from build123d import *

# Parameters (mm, degrees)
SKETCH1_W           = 82.48
SKETCH1_H           = 33
BOSS_EXTRUDE1_DEPTH = 5
SKETCH2_W           = 82.48
SKETCH2_H           = 5
BOSS_EXTRUDE2_DEPTH = 5
CHAMFER1_SIZE       = 5
CUT_EXTRUDE1_REACH  = 92.95
SKETCH3_R           = 5.35
BOSS_EXTRUDE3_DEPTH = 22
SKETCH5_W           = 21.546115959
SKETCH5_H           = 2.75
SKETCH5_W_2         = 39.193884041
BOSS_EXTRUDE4_DEPTH = 15
SKETCH6_W           = 4
SKETCH6_H           = 23
BOSS_EXTRUDE5_DEPTH = 3
CUT_EXTRUDE2_REACH  = 95.44
SKETCH7_W           = 20.522158998
SKETCH7_H           = 19


with BuildPart() as part:
    # Sketch1 → Boss-Extrude1 (new body)
    with BuildSketch(Plane.XY):
        with Locations((41.24, 16.5)):
            Rectangle(SKETCH1_W, SKETCH1_H)
    extrude(amount=BOSS_EXTRUDE1_DEPTH)

    # Sketch2 → Boss-Extrude2 (add)
    with BuildSketch(Plane(origin=(0, 33, 0), x_dir=(1, 0, 0), z_dir=(0, 1, 0))):
        with Locations((41.24, -2.5)):
            Rectangle(SKETCH2_W, SKETCH2_H)
    extrude(amount=BOSS_EXTRUDE2_DEPTH)

    # Chamfer1
    chamfer1_edges = [part.edges().sort_by_distance(p)[0] for p in [
        (0, 38, 2.5),
        (82.48, 38, 2.5),
    ]]
    chamfer(chamfer1_edges, length=CHAMFER1_SIZE)

    # Sketch3 → Cut-Extrude1 (cut, up to next)
    with BuildSketch(Plane.XY.offset(5), mode=Mode.PRIVATE) as cut_extrude1_sk1:
        with Locations((62.98, 20)):
            Circle(SKETCH3_R)
    cut_extrude1_tool1 = extrude(cut_extrude1_sk1.sketch, amount=-CUT_EXTRUDE1_REACH, mode=Mode.PRIVATE) & part.part
    add(cut_extrude1_tool1.solids().sort_by_distance((62.98, 20, 5))[0], mode=Mode.SUBTRACT)

    # Sketch4 → Boss-Extrude3 (add)
    with BuildSketch(Plane(origin=(0, 0, 0), x_dir=(-1, 0, 0), z_dir=(0, 0, -1))):
        Polygon((-82.48, 33), (0, 33), (-5, 38), (-77.48, 38), align=None)
    extrude(amount=BOSS_EXTRUDE3_DEPTH)

    # Sketch5 → Boss-Extrude4 (add)
    with BuildSketch(Plane(origin=(0, 0, 0), x_dir=(-1, 0, 0), z_dir=(0, 0, -1))):
        Polygon((-79.23, 33), (-77.73, 33), (-77.73, 29.75), (-75.73, 29.75), (-75.73, 28.25), (-81.23, 28.25), (-81.23, 29.75), (-79.23, 29.75), align=None)
        Polygon((-6.49, 33), (-4.99, 33), (-4.99, 29.75), (-2.99, 29.75), (-2.99, 28.25), (-8.49, 28.25), (-8.49, 29.75), (-6.49, 29.75), align=None)
        with Locations((-68.456942021, 4.625)):
            Rectangle(SKETCH5_W, SKETCH5_H)
        with Locations((-22.586942021, 4.625)):
            Rectangle(SKETCH5_W_2, SKETCH5_H)
    extrude(amount=BOSS_EXTRUDE4_DEPTH)

    # Sketch6 → Boss-Extrude5 (add)
    with BuildSketch(Plane(origin=(0, 0, 0), x_dir=(-1, 0, 0), z_dir=(0, 0, -1))):
        with Locations((-49.262158998, 21.5)):
            Rectangle(SKETCH6_W, SKETCH6_H)
        with Locations((-38.262158998, 21.5)):
            Rectangle(SKETCH6_W, SKETCH6_H)
    extrude(amount=BOSS_EXTRUDE5_DEPTH)

    # Sketch7 → Cut-Extrude2 (cut, up to next)
    with BuildSketch(Plane(origin=(0, 0, 0), x_dir=(-1, 0, 0), z_dir=(0, 0, -1)), mode=Mode.PRIVATE) as cut_extrude2_sk1:
        with Locations((-19.751079499, 19.5)):
            Rectangle(SKETCH7_W, SKETCH7_H)
    cut_extrude2_tool1 = extrude(cut_extrude2_sk1.sketch, amount=-CUT_EXTRUDE2_REACH, mode=Mode.PRIVATE) & part.part
    add(cut_extrude2_tool1.solids().sort_by_distance((19.751079, 19.5, 0))[0], mode=Mode.SUBTRACT)


solid = part.part
Here's how the part is built. I have some questions about the finished solid (model axes, mm). A direction names the side the tool comes from. Give positions to 0.01 mm unless a question says otherwise; leave off trailing zeros. Order: outer loops, then holes, each group sorted by start corner. A loop starts at its lowest first (then second) coordinate and runs counter-clockwise, first axis right, second up. Notation, with made-up numbers: (71, 65.25) -> (85, 65.25) arc R15 ccw to (85, 75.25) -> close; hole circle Ø1 at (-4.75, -13). An arc over 180 degrees is marked (long way). One line per item, written item: value. Start each with the question number.
1. We'd pull the mould along X, two halves only. Please class faces 1 (the face through (42, 33, -11)), 2 (the face through (69, 3.25, -7)), 3 (the face through (4.99, 31, -7)): released by +X, released by -X, zero draft, split by the parting line, or undercut.
2. Imagine slicing it at D-D, the plane y = 26.5. List the corners of the cut face in (x, z) for me, plus the area to 3 significant figures.
3. I need wall thicknesses on probe 1 along Y at (x, z) = (8, -7.25); probe 2 along Y at (x, z) = (62.98, 1.7); probe 3 along X at (y, z) = (17.5, 3.75). Which ranges of each line are inside material? Lowest first, please. Write a range as from..to.
4. Imagine slicing it at B-B, the plane y = 20. List the corners of the cut face in (x, z) for me.
5. Imagine slicing it at C-C, the plane x = 28. List the corners of the cut face in (y, z) for me.
6. For faces 4 (the face through (6.49, 31, -7)), 5 (the face through (78, 28.25, -7)), 6 (the face through (23, 5, -15)), 7 (the face through (69, 6, -7)), 8 (the face through (9.49, 19, 2)), which set-ups out of +Z, -Z, +X, -X, +Y, -Y let a thin tool reach every point of the face, with its end or its side?
7. Imagine slicing it at A-A, the plane z = -13.25. List the corners of the cut face in (x, y) for me.
8. Will these pins go through, and if not, where does the flat tip stop? pin 1 Ø4 at (x, y) = (7, 30) entering from -Z; pin 2 Ø1.5 at (x, z) = (39, -2) entering from -Y; pin 3 Ø3 at (x, y) = (31, 18) entering from -Z.
Values follow:
1. face 1: undercut
1. face 2: zero draft
1. face 3: released by -X
2. outline: (0, 0) -> (9.49, 0) -> (9.49, 5) -> (0, 5) -> close; (30.01, 0) -> (36.26, 0) -> (36.26, -3) -> (40.26, -3) -> (40.26, 0) -> (47.26, 0) -> (47.26, -3) -> (51.26, -3) -> (51.26, 0) -> (82.48, 0) -> (82.48, 5) -> (30.01, 5) -> close
2. area: 334 mm2
3. probe 1: y = 3.25..6, 28.25..29.75, 33..38
3. probe 2: y = 0..14.65, 25.35..38
3. probe 3: x = 0..9.49, 30.01..58.25, 67.71..82.48
4. outline: (0, 0) -> (9.49, 0) -> (9.49, 5) -> (0, 5) -> close; (30.01, 0) -> (36.26, 0) -> (36.26, -3) -> (40.26, -3) -> (40.26, 0) -> (47.26, 0) -> (47.26, -3) -> (51.26, -3) -> (51.26, 0) -> (57.63, 0) -> (57.63, 5) -> (30.01, 5) -> close; (68.33, 0) -> (82.48, 0) -> (82.48, 5) -> (68.33, 5) -> close
5. outline: (0, 0) -> (3.25, 0) -> (3.25, -15) -> (6, -15) -> (6, 0) -> (10, 0) -> (10, 5) -> (0, 5) -> close; (29, 0) -> (33, 0) -> (33, -22) -> (38, -22) -> (38, 5) -> (29, 5) -> close
6. face 4: -Z
6. face 5: -Z, +X
6. face 6: -Z, +X, -X, -Y
6. face 7: -Z, +X, -X
6. face 8: +Z, -Z
7. outline: (0, 33) -> (4.99, 33) -> (4.99, 29.75) -> (2.99, 29.75) -> (2.99, 28.25) -> (8.49, 28.25) -> (8.49, 29.75) -> (6.49, 29.75) -> (6.49, 33) -> (77.73, 33) -> (77.73, 29.75) -> (75.73, 29.75) -> (75.73, 28.25) -> (81.23, 28.25) -> (81.23, 29.75) -> (79.23, 29.75) -> (79.23, 33) -> (82.48, 33) -> (77.48, 38) -> (5, 38) -> close; (2.99, 3.25) -> (42.18, 3.25) -> (42.18, 6) -> (2.99, 6) -> close; (57.68, 3.25) -> (79.23, 3.25) -> (79.23, 6) -> (57.68, 6) -> close
8. pin 1: stops at z = -15
8. pin 2: stops at y = 3.25
8. pin 3: stops at z = 0
